Could you check a few things on this drawing? It's one solid part, dimensions in mm from its lowest x, y, z. Coordinates: 2 decimals unless noted, no trailing zeros. Write each loop counter-clockwise with the first axis right and the second up, starting at its lowest first coordinate (ties: lowest second). Pieces come first, ordered by that corner, then holes.
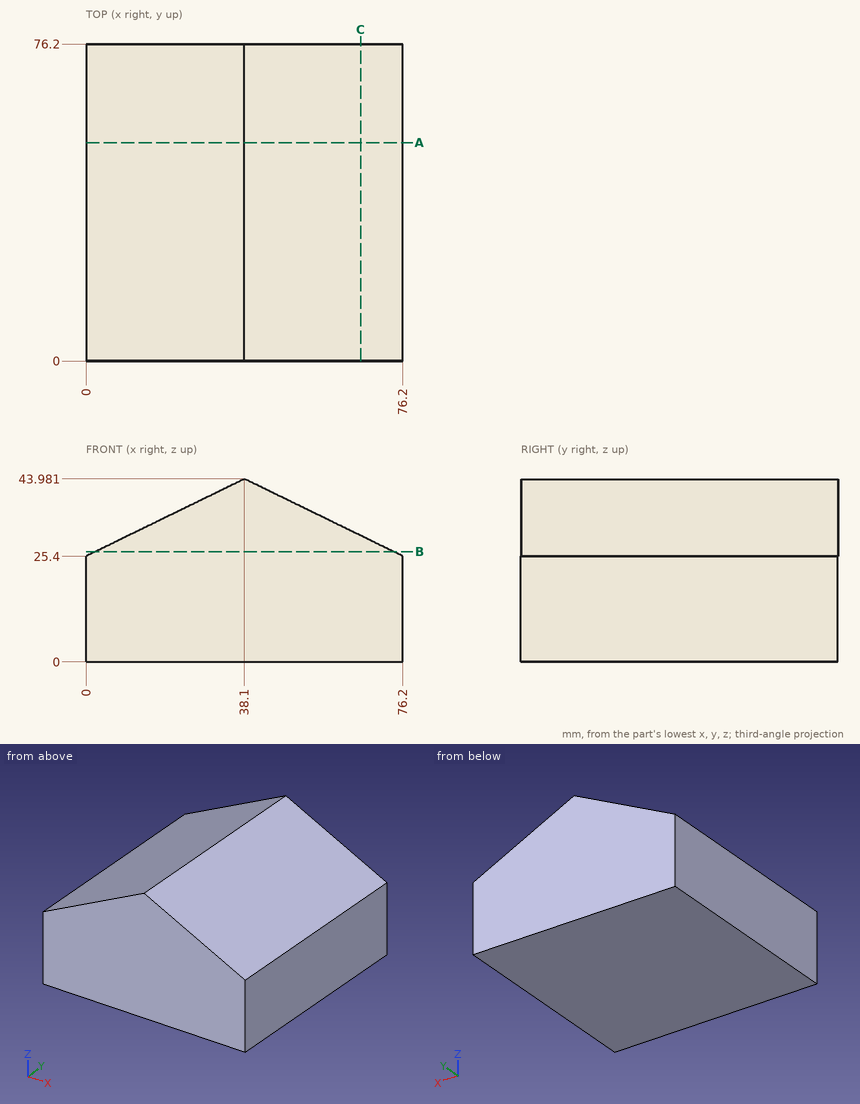
1) Imagine slicing it at C-C on x = 66. Please give me the cut outline in (y, z), then the cut area to 3 significant figures.
Values follow:
outline: (0, 0) - (76.2, 0) - (76.2, 30.37) - (0, 30.37) - close
area: 2,310 mm2
2) I need wall thicknesses on probe 1 along X at (y, z) = (42.5, 26); probe 2 along Z at (x, y) = (73, 5.5); probe 3 along Z at (x, y) = (29, 19.5). Which ranges of each line are inside material? Lowest first, please.
Values follow:
probe 1: x = 1.23 to 74.97
probe 2: z = 0 to 26.96
probe 3: z = 0 to 39.54
3) Imagine slicing it at A-A on y = 52.5. Please give me the cut outline in (x, z), then the cut area to 3 significant figures.
Values follow:
outline: (0, 0) - (76.2, 0) - (76.2, 25.4) - (38.1, 43.98) - (0, 25.4) - close
area: 2,640 mm2
4) Will these pins go through, and if not, where does the flat tip stop? pin 1 (3 mm diameter, centred on x = 25.5, y = 68.5, fed in from +Z); pin 2 (12 mm diameter, centred on x = 17, y = 42, fed in from +Z).
Values follow:
pin 1: stops at z = 38.57
pin 2: stops at z = 36.62
5) Imagine slicing it at B-B on z = 26.5. Please give me the cut outline in (x, y).
Values follow:
outline: (2.26, 0) - (73.94, 0) - (73.94, 76.2) - (2.26, 76.2) - close
